For this review, take the finished solid that the model builds, in its own axes (mm). A direction names the side the tool comes from. Give positions to 0.01 mm unless a question says otherwise; leave off trailing zeros. Order: outer loops, then holes, each group sorted by start corner. A loop starts at its lowest first (then second) coordinate and runs counter-clockwise, first axis right, second up.
from build123d import *

# Parameters (mm, degrees)
SKETCH1_W            = 38
SKETCH1_H            = 124
BOSS_EXTRUDE1_DEPTH  = 35
SKETCH2_R            = 15
BOSS_EXTRUDE2_DEPTH  = 34
FILLET1_R            = 5
SKETCH3_R            = 11
CUT_EXTRUDE1_DEPTH   = 1000
SKETCH5_W            = 24.830906905
SKETCH5_H            = 111.203932215
BOSS_EXTRUDE3_DEPTH  = 30
SKETCH6_W            = 60
SKETCH6_H            = 100
BOSS_EXTRUDE4_DEPTH  = 30
CUT_EXTRUDE5_DEPTH   = 100
SKETCH10_R           = 7.5
CUT_EXTRUDE6_DEPTH   = 10
SKETCH11_R           = 2.301516645
CUT_EXTRUDE7_DEPTH   = 10
LPATTERN1_COUNT      = 2
LPATTERN1_PITCH      = 25
LPATTERN1_COUNT_DIR2 = 2
LPATTERN1_PITCH_DIR2 = 25
SKETCH4_R            = 9
CUT_EXTRUDE_1_DEPTH  = 17


with BuildPart() as part:
    # Sketch1 → Boss-Extrude1 (new body)
    with BuildSketch(Plane.XY):
        with Locations((-7.18125, -12.690625)):
            Rectangle(SKETCH1_W, SKETCH1_H)
    extrude(amount=BOSS_EXTRUDE1_DEPTH)

    # Sketch2 → Boss-Extrude2 (add)
    with BuildSketch(Plane.XY.offset(35)):
        with Locations((-23.18125, -34.690625)):
            Circle(SKETCH2_R)
    extrude(amount=-BOSS_EXTRUDE2_DEPTH)

    # Fillet1
    fillet1_edges = [part.edges().sort_by_distance(p)[0] for p in [
        (-26.18125, -19.993686543, 18),
        (-26.18125, -49.387563457, 18),
    ]]
    fillet(fillet1_edges, radius=FILLET1_R)

    # Sketch3 → Cut-Extrude1 (cut)
    with BuildSketch(Plane.XZ.offset(74.690625)):
        with Locations((-7.18125, 18)):
            Circle(SKETCH3_R)
    extrude(amount=-CUT_EXTRUDE1_DEPTH, mode=Mode.SUBTRACT)

    # Sketch5 → Boss-Extrude3 (add)
    with BuildSketch(Plane(origin=(0, 0, 0), x_dir=(-1, 0, 0), z_dir=(0, 0, -1))):
        with Locations((5.153648801, -6.911017359)):
            Rectangle(SKETCH5_W, SKETCH5_H)
    extrude(amount=BOSS_EXTRUDE3_DEPTH)

    # Sketch6 → Boss-Extrude4 (add)
    with BuildSketch(Plane(origin=(0, 0, -30), x_dir=(-1, 0, 0), z_dir=(0, 0, -1))):
        with Locations((6.18125, -0.690625)):
            Rectangle(SKETCH6_W, SKETCH6_H)
    extrude(amount=BOSS_EXTRUDE4_DEPTH)

    # Sketch9 → Cut-Extrude5 (cut)
    with BuildSketch(Plane(origin=(7.261804652, 0, 0), x_dir=(0, 0, -1), z_dir=(1, 0, 0))):
        Polygon((0, 52.602660234), (0, 31.309375), (30, 39.309375), (30, 52.602660234), align=None)
        Polygon((0, -56.690625), (0, -66.373805341), (30, -69.28142928), (30, -44.690625), align=None)
    extrude(amount=-CUT_EXTRUDE5_DEPTH, mode=Mode.SUBTRACT)

    # Sketch10 → Cut-Extrude6 (cut)
    with BuildSketch(Plane.ZY.offset(36.18125)):
        with Locations((-45, -15.690625)):
            Circle(SKETCH10_R)
    extrude(amount=-CUT_EXTRUDE6_DEPTH, mode=Mode.SUBTRACT)

    # Sketch11 → Cut-Extrude7 (cut)
    with BuildSketch(Plane(origin=(0, 49.309375, 0), x_dir=(1, 0, 0), z_dir=(0, 1, 0))):
        with Locations((6.624715973, -28.639015413)):
            Circle(SKETCH11_R)
    cut_extrude7 = extrude(amount=-CUT_EXTRUDE7_DEPTH, mode=Mode.SUBTRACT)

    # LPattern1: Cut-Extrude7 2 × 2
    with Locations(*[(-i * LPATTERN1_PITCH, 0, -j * LPATTERN1_PITCH_DIR2) for i in range(LPATTERN1_COUNT) for j in range(LPATTERN1_COUNT_DIR2) if (i, j) != (0, 0)]):
        add(cut_extrude7, mode=Mode.SUBTRACT)

    # Sketch4 → Вырез-Вытянуть1 (cut)
    with BuildSketch(Plane.XY.offset(35)):
        with Locations((-23.18125, -34.690625)):
            Circle(SKETCH4_R)
    extrude(amount=-CUT_EXTRUDE_1_DEPTH, mode=Mode.SUBTRACT)


solid = part.part
1) We need section A-A on z = -45. Give the boundary of the cut face in (x, y), then the cut area to 3 significant figures.
Answer sheet:
outline: (-36.18, -50.69) - (23.82, -50.69) - (23.82, 49.31) - (-36.18, 49.31) - (-36.18, -8.19) - (-26.18, -8.19) - (-26.18, -23.19) - (-36.18, -23.19) - close
area: 5,850 mm2
2) We need section B-B on y = -65.5. Give the boundary of the cut face in (x, z), then the cut area to 3 significant figures.
Answer sheet:
outline: (-26.18, 0) - (11.82, 0) - (11.82, 35) - (-26.18, 35) - close; hole circle Ø22 at (-7.18, 18)
area: 950 mm2
3) To check wall thickness, follow line 1 (Z direction, x = -19, y = -21); line 2 (Z direction, x = 21.5, y = 13.5); line 3 (Z direction, x = -27, y = -42). State the ranges of each line that lie inside material, in increasing order.
Answer sheet:
line 1: z = -60 to -30, 0 to 35
line 2: z = -60 to -30
line 3: z = -60 to -30, 1 to 18
4) Tool access review of faces 1 (the face through (-18, 39.309, 4)), 2 (the face through (-26.181, -16, -45)), 3 (the face through (-20, -12, 0)), 4 (the face through (-17.569, -9, -15)): name each direction out of +Z, -Z, +X, -X, +Y, -Y from which nothing blocks a thin tool from reaching the whole face with its end or side.
Answer sheet:
face 1: +Y
face 2: -X
face 3: none
face 4: -X, +Y, -Y
5) Draft analysis for pull direction Z (two halves, no side actions). For faces 5 (the face through (-18, 39.309, 29)), 6 (the face through (11.819, -14, 17)), 7 (the face through (-8, -12, 35)), state which applies: +Z half, -Z half, draft (parallel to the pull), parting line (faces both ways), or undercut.
Answer sheet:
face 5: undercut
face 6: draft
face 7: +Z half
6) We need section D-D on x = 14.5. Give the boundary of the cut face in (y, z), then the cut area to 3 significant figures.
Answer sheet:
outline: (-50.69, -60) - (49.31, -60) - (49.31, -30) - (-50.69, -30) - close
area: 3,000 mm2
7) We need section C-C on z = 20. Give the boundary of the cut face in (x, y).
Answer sheet:
outline: (-29.18, -48.44) arc R5 cw to (-26.18, -53.02) - (-26.18, -74.69) - (-18, -74.69) - (-18, -42.05) arc R9 cw (long way) to (-18, -27.33) - (-18, 49.31) - (-26.18, 49.31) - (-26.18, -16.36) arc R5 cw to (-29.18, -20.94) arc R15 ccw to start; (3.64, -74.69) - (11.82, -74.69) - (11.82, 49.31) - (3.64, 49.31) - close
8) Clearance check with flat-ended pins moving along their axes: pin 1 (1.4 mm diameter, centred on x = -19, z = 28.5, fed in from +Y); pin 2 (24 mm diameter, centred on y = -0.5, z = -13.5, fed in from -X); pin 3 (15 mm diameter, centred on x = -3.5, z = -51.5, fed in from -Y). State where each tip first meets the part, or that it passes through.
Answer sheet:
pin 1: stops at y = 39.31
pin 2: stops at x = -17.57
pin 3: stops at y = -50.69
